The figure shows three views and two pictorial views of one solid part (mm, origin at its lowest corner). Answer the questions. A direction names the side the tool comes from. Coordinates: 2 decimals unless noted, no trailing zeros. Write each loop counter-clockwise with the first axis right and the second up, starting at its lowest first coordinate (ties: lowest second). Pieces come first, ordered by that corner, then holes.
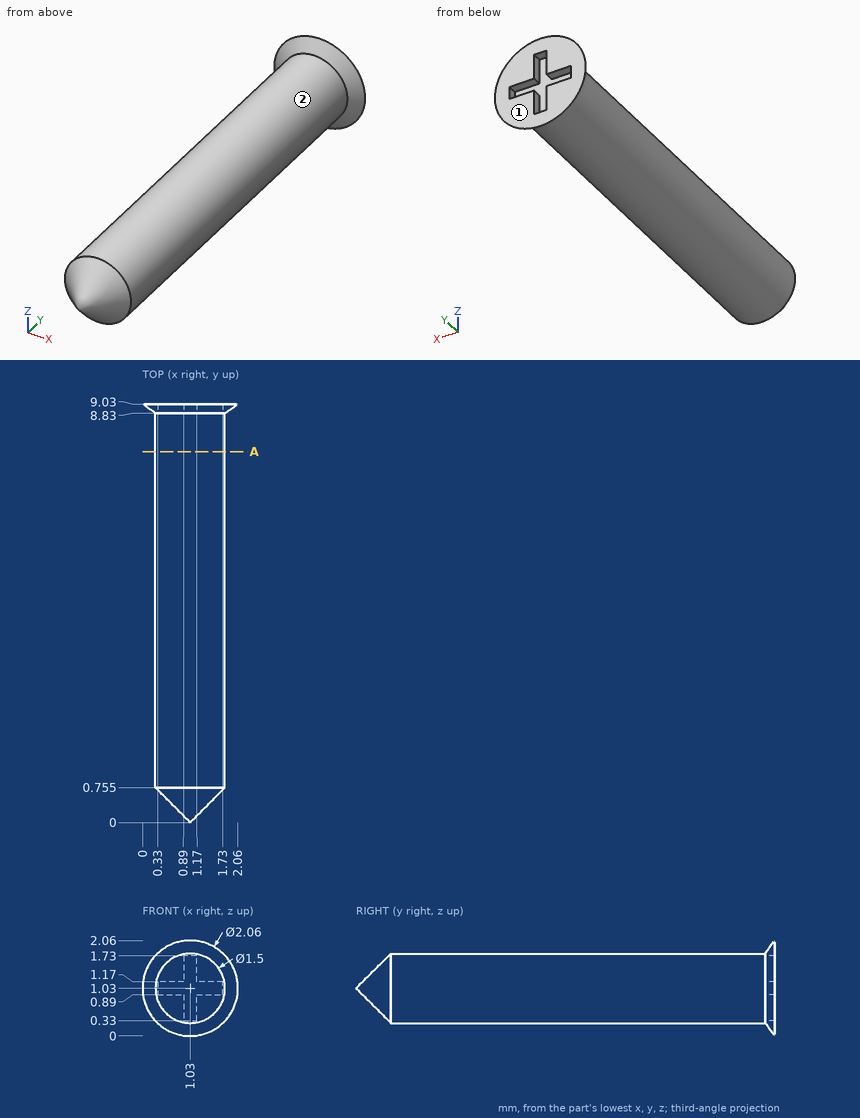
1. Section A-A on y = 8 is taken. Give the vertices of the cut face in (x, z).
Results found:
outline: circle Ø1.5 at (1.03, 1.03)
2. A tool of negligible diameter and unlimited length cuts with its end or side. For the marked faces 1 and 2, from which of +Z, -Z, +X, -X, +Y, -Y can it reach the whole face along a straight path? Write none if from no direction.
Results found:
face 1: +Z, -Z, +X, -X, +Y
face 2: -Y
3. Find the intervals of material crossed by L1, parallel to X at y = 3.75, z = 1.3; L2, parallel to Z at x = 1, y = 5; L3, parallel to X at y = 2, z = 1.5 (1 decimal), in increasing order.
Results found:
L1: x = 0.33 to 1.73
L2: z = 0.28 to 1.78
L3: x = 0.4 to 1.6
4. A flat-ended cylindrical pin translates along its axis: P1, Ø1, axis at x = 0.5, y = 5, coming from the -Z side. Find the tip coordinate at first contact, or state that the pin passes through.
Results found:
P1: stops at z = 0.28
